```python
from build123d import *

# Parameters (mm, degrees)
SKETCH1_W                      = 33
SKETCH1_H                      = 11
SKETCH1_W_2                    = 30
SKETCH1_H_2                    = 8
BOSS_EXTRUDE1_DEPTH            = 8
SKETCH3_R                      = 0.8
CUT_EXTRUDE3_DEPTH             = 22.38340478
CUT_EXTRUDE5_REACH             = 21.144
SKETCH5_R                      = 3.5
CUT_EXTRUDE5_DIRECTION_2_DEPTH = 20.144189719
CUT_EXTRUDE4_DEPTH             = 22.38340478
CUT_EXTRUDE9_START             = -1.5
CUT_EXTRUDE9_DEPTH             = 8
SKETCH9_W                      = 22
SKETCH9_H                      = 8
CUT_EXTRUDE8_DEPTH             = 2.25
BOSS_EXTRUDE8_START            = 2
SKETCH12_W                     = 28.108309096
SKETCH12_H                     = 11
SKETCH12_R                     = 3.5
BOSS_EXTRUDE8_DEPTH            = 2
FILLET1_R                      = 1
CHAMFER1_SIZE                  = 1.5
CHAMFER1_SIZE_2                = 3.369055161
CHAMFER2_SIZE                  = 0.5
CHAMFER2_SIZE2                 = 1.123018387
CHAMFER3_SIZE                  = 0.5
CHAMFER3_SIZE2                 = 1.123018387
BOSS_EXTRUDE9_REACH            = 20.168
HEAT_SHRINK_OFFSET_SCALE_SCALE = 1.03


with BuildPart() as part:
    # Sketch1 → Boss-Extrude1 (new body)
    # profile 1 of 2: a face of its own
    with BuildSketch(Plane(origin=(0, 0, 0), x_dir=(1, 0, 0), z_dir=(0, 1, 0))):
        Rectangle(SKETCH1_W, SKETCH1_H)
        Rectangle(SKETCH1_W_2, SKETCH1_H_2, mode=Mode.SUBTRACT)
    # profile 2 of 2: a face of its own
    with BuildSketch(Plane(origin=(0, 0, 0), x_dir=(1, 0, 0), z_dir=(0, 1, 0))):
        Rectangle(SKETCH1_W_2, SKETCH1_H_2)
    extrude(amount=BOSS_EXTRUDE1_DEPTH)

    # Sketch3 → Cut-Extrude3 (cut, through all)
    with BuildSketch(Plane.XY.offset(5.5)):
        with Locations((-12.5, 4)):
            Circle(SKETCH3_R)
        with Locations((12.5, 4)):
            Circle(SKETCH3_R)
    extrude(amount=-CUT_EXTRUDE3_DEPTH, mode=Mode.SUBTRACT)

    # Sketch5 → Cut-Extrude5 (cut, up to next)
    with BuildSketch(Plane(origin=(0, 8, 0), x_dir=(1, 0, 0), z_dir=(0, 1, 0)), mode=Mode.PRIVATE) as cut_extrude5_sk1:
        with Locations(Location((0, 0, 0), (0, 0, 90))):
            Circle(SKETCH5_R)
    cut_extrude5_tool1 = extrude(cut_extrude5_sk1.sketch, amount=-CUT_EXTRUDE5_REACH, mode=Mode.PRIVATE) & part.part
    add(cut_extrude5_tool1.solids().sort_by_distance((0, 8, 0))[0], mode=Mode.SUBTRACT)

    # Sketch5 → Cut-Extrude5 direction 2 (cut)
    with BuildSketch(Plane(origin=(0, 8, 0), x_dir=(1, 0, 0), z_dir=(0, 1, 0))):
        with Locations(Location((0, 0, 0), (0, 0, 90))):
            Circle(SKETCH5_R)
    extrude(amount=CUT_EXTRUDE5_DIRECTION_2_DEPTH, mode=Mode.SUBTRACT)

    # Sketch4 → Cut-Extrude4 (cut, through all)
    with BuildSketch(Plane.XY.offset(5.5)):
        Polygon((-16.5, 0), (-14.054154548, 8), (-16.5, 8), align=None)
        Polygon((16.5, 0), (14.054154548, 8), (16.5, 8), align=None)
    extrude(amount=-CUT_EXTRUDE4_DEPTH, mode=Mode.SUBTRACT)

    # Sketch14 → Cut-Extrude9 (cut)
    with BuildSketch(Plane.XY.offset(5.5).offset(CUT_EXTRUDE9_START)):
        Polygon((-15, 0), (15, 0), (14.235673296, 2.5), (-14.235673296, 2.5), align=None)
    extrude(amount=-CUT_EXTRUDE9_DEPTH, mode=Mode.SUBTRACT)

    # Sketch9 → Cut-Extrude8 (cut)
    with BuildSketch(Plane.XZ.offset(-2.5)):
        Rectangle(SKETCH9_W, SKETCH9_H)
    extrude(amount=-CUT_EXTRUDE8_DEPTH, mode=Mode.SUBTRACT)

    # Sketch12 → Boss-Extrude8 (add)
    with BuildSketch(Plane(origin=(0, 8, 0), x_dir=(1, 0, 0), z_dir=(0, 1, 0)).offset(BOSS_EXTRUDE8_START)):
        Rectangle(SKETCH12_W, SKETCH12_H)
        with Locations(Location((0, 0, 0), (0, 0, 90))):
            Circle(SKETCH12_R, mode=Mode.SUBTRACT)
    extrude(amount=-BOSS_EXTRUDE8_DEPTH)

    # Fillet1
    fillet1_edges = [part.edges().sort_by_distance(p)[0] for p in [
        (0, 10, 5.5),
        (0, 10, -5.5),
    ]]
    fillet(fillet1_edges, radius=FILLET1_R)

    # Chamfer1
    # the kernel refuses this chamfer: 3.369055161, 1.5 mm, written as the material it takes off along each edge
    with BuildSketch(Plane(origin=(0, 4.75, 0), x_dir=(0, 0, -1), z_dir=(1, 0, 0))) as chamfer1_piece_1_section:
        Polygon((3.5, CHAMFER1_SIZE), (3.5 + CHAMFER1_SIZE_2, 0), (3.5, 0), align=None)
    chamfer1_piece_1 = revolve(axis=Axis((0, 4.75, 0), (0, 1, 0)), mode=Mode.PRIVATE)
    chamfer1_piece_1 = split(chamfer1_piece_1, bisect_by=Plane(origin=(-3.432540166, 6.000877118, 4), z_dir=(0, 0, -1)), keep=Keep.TOP, mode=Mode.PRIVATE)
    chamfer1_piece_1 = split(chamfer1_piece_1, bisect_by=Plane(origin=(-3.432540166, 6.000877118, -4), z_dir=(0, 0, 1)), keep=Keep.TOP, mode=Mode.PRIVATE)
    add(chamfer1_piece_1, mode=Mode.SUBTRACT)

    # Chamfer2
    chamfer2_edges = [part.edges().sort_by_distance(p)[0] for p in [
        (-11, 2.5, 0),
    ]]
    chamfer2_side = [part.faces().sort_by_distance(p)[0] for p in [
        (-11, 3.625, 0),
    ]]
    chamfer(chamfer2_edges, length=CHAMFER2_SIZE, length2=CHAMFER2_SIZE2, reference=chamfer2_side[0])

    # Chamfer3
    chamfer3_edges = [part.edges().sort_by_distance(p)[0] for p in [
        (11, 2.5, 0),
    ]]
    chamfer3_side = [part.faces().sort_by_distance(p)[0] for p in [
        (11, 3.625, 0),
    ]]
    chamfer(chamfer3_edges, length=CHAMFER3_SIZE, length2=CHAMFER3_SIZE2, reference=chamfer3_side[0])

    # Sketch17 → Boss-Extrude9 (add, up to next)
    with BuildSketch(Plane.XZ.offset(-4.75), mode=Mode.PRIVATE) as boss_extrude9_sk1:
        Polygon((5.910492264, -3.5), (0, -3.5), (-5.910492264, -3.5), (-5.910492264, -4), (5.910492264, -4), align=None)
    boss_extrude9_tool1 = extrude(boss_extrude9_sk1.sketch, amount=-BOSS_EXTRUDE9_REACH, mode=Mode.PRIVATE) - part.part
    add(boss_extrude9_tool1.solids().sort_by_distance((0, 4.75, -3.75))[0])


with BuildPart() as part_1:
    # Heat shrink offset scale: scaled about (0, 5.8657217, -0.009275667)
    add(part.part.scale(HEAT_SHRINK_OFFSET_SCALE_SCALE).moved(Location((0, -0.175971651, 0.00027827))))


solid = part_1.part
```
Part model, mm, in its own coordinate system. A direction names the side the tool comes from. Coordinates: 2 decimals unless noted, no trailing zeros. Loops run counter-clockwise (first coordinate to the right, second up) from the corner with the lowest first, then second, coordinate; pieces in that order, holes last. Notation, with made-up numbers: (82, -15.75) - (136, -15.75) arc R29 cw to (136, 17.25) - close; hole circle Ø7 at (55, 47.5). An arc over 180 degrees is marked (long way). Write item = value, one per line. Start each with the question number.
Item 1: Cut at C-C, the plane z = 0.25. State how many separate pieces and enclosed holes the cut face has, and give its area (3 significant figures).
Item 2: Cut at B-B, the plane y = 2. Give the cut face in (x, z).
Item 3: 3-axis set-ups, long thin cutter, end or side, ignore diameter. For faces 5 (the flat face through (0, 2, -4.12)), 6 (the cylindrical face through (13.318, 4.639, 0.08)), 7 (the flat face through (14.476, 9, 0)), 8 (the flat face through (-14.476, 9, 0)): which of +Z, -Z, +X, -X, +Y, -Y reach the whole face in a straight line?
Item 4: Cut at A-A, the plane x = 14. Give the cut face in (y, z).
Item 5: Mould opens along Z. For faces 1 (the flat face through (-14, 2.399, 0)), 2 (the cylindrical face through (0.203, 9.83, -5.355)), 3 (the flat face through (-11.33, 4, 0)), 4 (the flat face through (-15.75, 3.89, 0.08)) say: released by +Z, released by -Z, zero draft, split by the parting line, or undercut.
Item 6: Wall check: L1, parallel to Z at x = 11.5, y = 1; L2, parallel to Z at x = 0, y = 7.7; L3, parallel to X at y = 9.5, z = -4. Give the ranges that are in metal, low to high. Write a range as from..to.
Item 7: Cut at D-D, the plane x = -10. Give the cut face in (y, z), and give its area (3 significant figures).
Item 8: Flat gauge pins, fed straight in: pin 1 Ø1.1 at (x, z) = (-14, 0.5) entering from -Y; pin 2 Ø2 at (x, y) = (12.88, 3.94) entering from -Z; pin 3 Ø0.5 at (y, z) = (3.5, -0.5) entering from -X; pin 4 Ø1 at (y, z) = (2.5, -0.5) entering from -X. Where does each tip first touch, or does it go through?
The answers:
q1.separate_pieces = 2
q1.enclosed_holes = 2
q1.area = 140 mm2
q2.outline = (-16.33, -5.66) - (16.33, -5.66) - (16.33, 5.67) - (-16.33, 5.67) - close; hole (-14.78, -4.12) - (14.78, -4.12) - (14.78, 4.12) - (-14.78, 4.12) - close
q3.face_5 = -Y
q3.face_6 = +Z, -Z
q3.face_7 = +Z, -Z, +X, +Y
q3.face_8 = +Z, -Z, -X, +Y
q4.outline = (-0.18, -5.66) - (9.09, -5.66) arc R1.03 ccw to (10.12, -4.63) - (10.12, 4.64) arc R1.03 ccw to (9.09, 5.67) - (-0.18, 5.67) - (-0.18, 4.12) - (2.4, 4.12) - (2.4, -4.12) - (-0.18, -4.12) - close
q5.face_1 = undercut
q5.face_2 = released by -Z
q5.face_3 = undercut
q5.face_4 = zero draft
q6.L1 = -5.66..-4.12, 4.12..5.67
q6.L2 = -5.66..-3.6, 3.61..5.67
q6.L3 = -14.48..14.48
q7.outline = (-0.18, -5.66) - (9.09, -5.66) arc R1.03 ccw to (10.12, -4.63) - (10.12, 4.64) arc R1.03 ccw to (9.09, 5.67) - (-0.18, 5.67) - (-0.18, 4.12) - (4.72, 4.12) - (4.72, -4.12) - (-0.18, -4.12) - close
q7.area = 75.9 mm2
q8.pin_1 = 2.4
q8.pin_2 = -5.66
q8.pin_3 = -15.95
q8.pin_4 = -16.33
